Part model, mm, in its own coordinate system. Face numbers are marked on the shaded views. A direction names the side the tool comes from. Coordinates: 2 decimals unless noted, no trailing zeros. Order: outer loops, then holes, each group sorted by start corner. A loop starts at its lowest first (then second) coordinate and runs counter-clockwise, first axis right, second up.
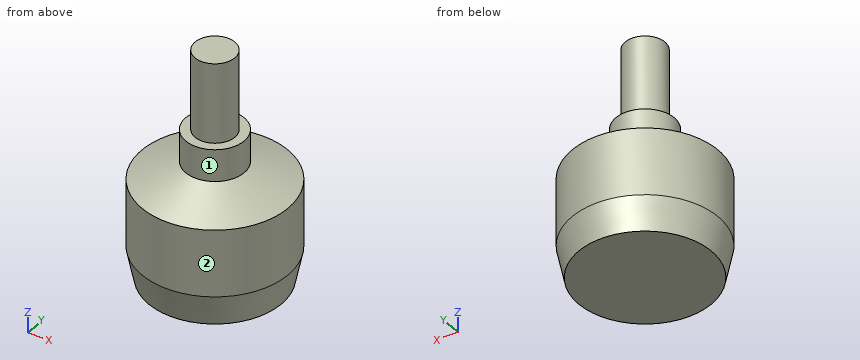
```python
from build123d import *

# Parameters (mm, degrees)
F1_START    = 6
F0_R        = 13.75
F0_R_2      = 12.5
F0_R_3      = 5.5
F0_R_4      = 3.75
F1_DEPTH    = 12.5
F2_DEPTH    = 22
F3_DEPTH    = 28
F4_DEPTH    = 7
F5_SIZE2    = 1.24999
F5_SIZE     = 5.99999
F6_S5_R     = 13.75
F6_T6_DEPTH = 21
F7_DEPTH    = 43


# Not quite as in the source:
# - a fillet or chamfer that OpenCascade refuses, or shapes differently, is made with other operations: its cross-section is extruded or revolved along the edge and cut away or added
# - a fillet or chamfer is up to 0.001 mm smaller than in the source, because OpenCascade refuses the exact size


with BuildPart() as f1:
    # F0 (on Top) → F1 (new body)
    with BuildSketch(Plane.XY.offset(F1_START)):
        Circle(F0_R)
        Circle(F0_R_2, mode=Mode.SUBTRACT)
        Circle(F0_R_2)
        Circle(F0_R_3, mode=Mode.SUBTRACT)
        Circle(F0_R_3)
        Circle(F0_R_4, mode=Mode.SUBTRACT)
        Circle(F0_R_4)
    extrude(amount=F1_DEPTH)

    # F0 (on Top) → F2 (join)
    with BuildSketch(Plane.XY):
        Circle(F0_R_3)
        Circle(F0_R_4, mode=Mode.SUBTRACT)
        Circle(F0_R_4)
    extrude(amount=F2_DEPTH)

    # F0 (on Top) → F3 (join)
    with BuildSketch(Plane.XY):
        Circle(F0_R_3)
        Circle(F0_R_4, mode=Mode.SUBTRACT)
        Circle(F0_R_4)
    extrude(amount=F3_DEPTH)

    # F0 (on Top) → F4 (join)
    with BuildSketch(Plane.XY):
        Circle(F0_R_2)
        Circle(F0_R_3, mode=Mode.SUBTRACT)
    extrude(amount=F4_DEPTH)

    # F5 (size 6 and 1.25 in the source; OpenCascade refuses exactly that, so slightly less here)
    f5_edges = [f1.edges().sort_by_distance(p)[0] for p in [
        (-12.5, 0, 6),
    ]]
    f5_side = f1.faces().sort_by_distance((-12.5, 0, 3))[0]
    chamfer(f5_edges, length=F5_SIZE, length2=F5_SIZE2, reference=f5_side)

    # F6: chamfer of 8.5 x 3.5 on 1 edges, made by hand


with BuildPart() as f6_tool2:
    # F6_s3 → F6_t4 (revolve)
    with BuildSketch(Plane.XZ):
        Polygon((14, 18.5), (5.5, 22), (5.5, 18.5), align=None)
    revolve(axis=Axis((0, 0, 18.5), (0, 0, -1)))

    # F6_s5 → F6_t6 (intersect, symmetric)
    with BuildSketch(Plane.XY.offset(20.2)):
        Circle(F6_S5_R)
    extrude(amount=F6_T6_DEPTH, both=True, mode=Mode.INTERSECT)


with BuildPart() as f1_1:
    add(f1.part)

    # F6_t1: union F6_tool2
    add(f6_tool2.part)

    # F0 (on Top) → F7 (join)
    with BuildSketch(Plane.XY):
        Circle(F0_R_4)
    extrude(amount=F7_DEPTH)


solid = f1_1.part
```
(1) Drop flat-ended pins along their axis: pin 1 (6 mm diameter, centred on x = 11, z = 11.5, fed in from -Y); pin 2 (1.5 mm diameter, centred on y = 10, z = 5.5, fed in from -X); pin 3 (6 mm diameter, centred on y = -4.5, z = 15.5, fed in from +X). Give the stop position or say it passes through.
(2) Slice it at D-D, the plane z = 33. Give the cut face in (x, y), then the cut area to 3 significant figures.
(3) Slice it at C-C, the plane z = 10. Give the cut face in (x, y), then the cut area to 3 significant figures.
(4) Tool access for the marked faces 1 and 2: list every direction of +Z, -Z, +X, -X, +Y, -Y with a clear straight run to the whole face (end or side of a thin tool).
(5) Probe line 1 (Z direction, x = -0.5, y = 5); line 2 (X direction, y = -4.75, z = 15); line 3 (Y direction, x = 0.25, z = 38). List the from-to ranges inside material, lowest first.
Here are the results:
1. pin 1: stops at y = -11.18
1. pin 2: stops at x = -10.06
1. pin 3: stops at x = 13.67
2. outline: circle Ø7.5 at (0, 0)
2. area: 44.2 mm2
3. outline: circle Ø27.5 at (0, 0)
3. area: 594 mm2
4. face 1: +Z
4. face 2: +Z, -Z
5. line 1: z = 0 to 28
5. line 2: x = -12.9 to 12.9
5. line 3: y = -3.74 to 3.74
